Work out the finished part from the listing and answer in its coordinate system (mm). A direction names the side the tool comes from. Give positions to 0.01 mm unless a question says otherwise; leave off trailing zeros. Write each loop counter-clockwise with the first axis right and the second up, starting at its lowest first coordinate (ties: lowest second). Pieces come first, ordered by that corner, then holes. Notation, with made-up numbers: (66, -4.75) - (114, -4.75) arc R10 ccw to (114, -0.75) - close; hole circle Ø9 at (2, 89). An arc over 180 degrees is marked (long way). Write each question's results on one line, items separated by ' | '. Start each with the question number.
from build123d import *

# Parameters (mm, degrees)
BOSS_EXTRUDE1_DEPTH     = 101.6
SKETCH4_W               = 21.336
SKETCH4_H               = 46.355
BOSS_EXTRUDE2_DEPTH     = 22.225
CUT_EXTRUDE5_DEPTH      = 97.870805748
CUT_EXTRUDE5_DEPTH_BACK = 97.870805748
SKETCH8_R               = 2.38125
CUT_EXTRUDE6_DEPTH      = 120.305668348


with BuildPart() as part:
    # Sketch1 → Boss-Extrude1 (new body)
    with BuildSketch(Plane.XY):
        Polygon((0, 0), (25.4, 0), (25.4, 57.15), (0, 12.7), align=None)
    extrude(amount=-BOSS_EXTRUDE1_DEPTH)

    # Sketch4 → Boss-Extrude2 (add)
    with BuildSketch(Plane(origin=(21.809590146, 0, -29.461184826), x_dir=(-1, 0, 0), z_dir=(0, -1, 0))):
        with Locations((8.665090146, 21.338815174)):
            Rectangle(SKETCH4_W, SKETCH4_H)
    extrude(amount=BOSS_EXTRUDE2_DEPTH)

    # Sketch7 → Cut-Extrude5 (cut, two sides: drawn at the far end of the back side and taken through both)
    with BuildSketch(Plane(origin=(0, 0, -73.9775), x_dir=(-1, 0, 0), z_dir=(0, 0, -1)).offset(-CUT_EXTRUDE5_DEPTH_BACK)):
        with BuildLine():
            Line((-22.098, -197.012283842), (-22.098, -22.225))
            ThreePointArc((-22.098, -22.225), (-13.1445, -13.2715), (-4.191, -22.225))
            Line((-4.191, -22.225), (-4.191, -197.012283842))
            Line((-4.191, -197.012283842), (-4.191, -546.586851526))
            Line((-4.191, -546.586851526), (-22.098, -546.586851526))
            Line((-22.098, -546.586851526), (-22.098, -197.012283842))
        make_face()
    extrude(amount=CUT_EXTRUDE5_DEPTH + CUT_EXTRUDE5_DEPTH_BACK, mode=Mode.SUBTRACT)

    # Sketch8 → Cut-Extrude6 (cut, through all)
    with BuildSketch(Plane(origin=(25.4, 0, 0), x_dir=(0, 0, -1), z_dir=(1, 0, 0))):
        with Locations(Location((5.842, 52.324, 0), (0, 0, 90))):
            Circle(SKETCH8_R)
        with Locations(Location((5.842, 4.572, 0), (0, 0, 90))):
            Circle(SKETCH8_R)
        with Locations(Location((94.837878374, 4.572, 0), (0, 0, 90))):
            Circle(SKETCH8_R)
        with Locations(Location((94.837878374, 52.324, 0), (0, 0, 90))):
            Circle(SKETCH8_R)
    extrude(amount=-CUT_EXTRUDE6_DEPTH, mode=Mode.SUBTRACT)


solid = part.part
Q1. A cutting plane is placed at A-A, the plane y = 52. Write down the section's boundary in (x, z).
Q2. A tool of negligible diameter and unlimited length cuts with its end or side. For faces 4 (the flat face through (23.812, -11, -50)), 5 (the flat face through (2.477, -11, -50)), 6 (the flat face through (15, 23, -101.6)), 7 (the flat face through (13, -8, -73.977)), from which of +Z, -Z, +X, -X, +Y, -Y can it reach the whole face along a straight path? Write none if from no direction.
Q3. The mould has two halves that part along Y. Classify faces 1 (the cylindrical face through (13.341, -13.274, -50.476)), 2 (the flat face through (13, -8, -27.622)), 3 (the cylindrical face through (23.778, 49.945, -94.733)): pulls with the +Y half, pulls with the -Y half, needs draft (parallel to the pull), parting line crosses it, or undercut.
Q4. A cutting plane is placed at C-C, the plane y = 5.5. Write down the section's boundary in (x, z).
Q5. Consider L1, parallel to X at y = -13, z = -54; L2, parallel to Y at x = 19.75, z = -97; L3, parallel to Z at x = 22.25, y = -11. Determine where each line is inside the solid, lowest interval first.
Q6. A cutting plane is placed at B-B, the plane x = 16. Write down the section's boundary in (y, z).
Q7. Given pin 1 (6.5 mm diameter, centred on y = -7, z = -62, fed in from +X); pin 2 (6 mm diameter, centred on y = 52.32, z = -94.84, fed in from -X); pin 3 (3 mm diameter, centred on y = 52.324, z = -5.842, fed in from +X); pin 4 (2 mm diameter, centred on x = 22, y = -3.5, fed in from -Z), each flat-ended and moving along its own axis, determine where each tip first touches the part or whether it passes through.
Q8. A cutting plane is placed at D-D, the plane z = -81.5. Write down the section's boundary in (x, y).
Result:
1) outline: (22.46, -101.6) - (25.4, -101.6) - (25.4, -97.2) - (22.46, -97.2) - close; (22.46, -92.48) - (25.4, -92.48) - (25.4, -8.2) - (22.46, -8.2) - close; (22.46, -3.48) - (25.4, -3.48) - (25.4, 0) - (22.46, 0) - close
2) face 4: +Z, -Z, +X, -Y | face 5: +Z, -Z, -X, -Y | face 6: -Z, +X, -X, +Y, -Y | face 7: -Z, +X, -X, -Y
3) face 1: pulls with the -Y half | face 2: needs draft | face 3: undercut
4) outline: (0, -101.6) - (25.4, -101.6) - (25.4, -97.03) - (0, -97.03) - close; (0, -92.64) - (25.4, -92.64) - (25.4, -8.03) - (0, -8.03) - close; (0, -3.65) - (25.4, -3.65) - (25.4, 0) - (0, 0) - close
5) L1: x = 2.48 to 23.81 | L2: y = 0 to 3.57, 5.57 to 47.26 | L3: z = -73.98 to -27.62
6) outline: (-13.74, -73.98) - (0, -73.98) - (0, -101.6) - (40.7, -101.6) - (40.7, 0) - (0, 0) - (0, -27.62) - (-13.74, -27.62) - close; hole circle Ø4.76 at (4.57, -94.84); hole circle Ø4.76 at (4.57, -5.84)
7) pin 1: stops at x = 23.81 | pin 2: stops at x = 20.93 | pin 3: passes through | pin 4: stops at z = -73.98
8) outline: (0, 0) - (25.4, 0) - (25.4, 57.15) - (0, 12.7) - close
